```python
from build123d import *

# Parameters (mm, degrees)
SKETCH1_R           = 6.35
SKETCH1_W           = 38.1
SKETCH1_H           = 13.818872092
BOSS_EXTRUDE1_DEPTH = 12.7


with BuildPart() as part:
    # Sketch1 → Boss-Extrude1 (new body)
    # profile 1 of 2: a face of its own
    with BuildSketch(Plane.XY):
        with BuildLine():
            Line((129.803523023, 13.72866743), (129.803523023, 32.77866743))
            Line((129.803523023, 32.77866743), (104.403523023, 32.77866743))
            Line((104.403523023, 32.77866743), (89.290523023, 32.77866743))
            Line((89.290523023, 32.77866743), (51.190523023, 32.77866743))
            Line((51.190523023, 32.77866743), (44.078523023, 32.77866743))
            Line((44.078523023, 32.77866743), (42.173523023, 32.77866743))
            ThreePointArc((42.173523023, 32.77866743), (0.864344867, 49.889489273), (-16.246476977, 91.19866743))
            Line((-16.246476977, 91.19866743), (-16.246476977, 115.32866743))
            Line((-16.246476977, 115.32866743), (-18.528129693, 124.368857105))
            ThreePointArc((-18.528129693, 124.368857105), (-35.296476977, 134.37866743), (-52.064824261, 124.368857105))
            Line((-52.064824261, 124.368857105), (-54.346476977, 115.32866743))
            Line((-54.346476977, 115.32866743), (-54.346476977, 91.438289009))
            ThreePointArc((-54.346476977, 91.438289009), (-63.850433524, 50.845698757), (-90.386686587, 18.691214671))
            Line((-90.386686587, 18.691214671), (-171.948476977, -43.42133257))
            Line((-171.948476977, -43.42133257), (-87.747476977, -43.42133257))
            Line((-87.747476977, -43.42133257), (-87.747476977, -49.77133257))
            Line((-87.747476977, -49.77133257), (-61.229320991, -49.77133257))
            Line((-61.229320991, -49.77133257), (-16.694588765, -49.77133257))
            Line((-16.694588765, -49.77133257), (64.652523023, -49.77133257))
            Line((64.652523023, -49.77133257), (64.652523023, -43.42133257))
            Line((64.652523023, -43.42133257), (129.803523023, -43.42133257))
            Line((129.803523023, -43.42133257), (129.803523023, -24.37133257))
            Line((129.803523023, -24.37133257), (139.328523023, -24.37133257))
            Line((139.328523023, -24.37133257), (139.328523023, 13.72866743))
            Line((139.328523023, 13.72866743), (129.803523023, 13.72866743))
        make_face()
        with Locations((-35.296476977, 115.32866743)):
            Circle(SKETCH1_R, mode=Mode.SUBTRACT)
    # profile 2 of 2: a face of its own
    with BuildSketch(Plane.XY):
        with Locations((70.240523023, 39.688103476)):
            Rectangle(SKETCH1_W, SKETCH1_H)
    extrude(amount=BOSS_EXTRUDE1_DEPTH)


solid = part.part
```
For this review, take the finished solid that the model builds, in its own axes (mm). A direction names the side the tool comes from. Give positions to 0.01 mm unless a question says otherwise; leave off trailing zeros. Order: outer loops, then holes, each group sorted by start corner. A loop starts at its lowest first (then second) coordinate and runs counter-clockwise, first axis right, second up.
1) For faces 1 (the face through (47, 32.779, 6)), 2 (the face through (135, 13.729, 6)), 3 (the face through (-54.346, 104, 6)), 4 (the face through (129.804, -34, 6)), list the 3-axis set-ups (+Z, -Z, +X, -X, +Y, -Y) from which the entire face can be reached by the end or side of a thin tool; tool diameter is ignored.
2) Insertion check: pin 1 (4 mm diameter, centred on x = 71.5, z = 7.5, fed in from +Y); pin 2 (7 mm diameter, centred on x = 45, z = 8, fed in from +Y); pin 3 (3 mm diameter, centred on y = -45.5, z = 3.5, fed in from +X); pin 4 (11.5 mm diameter, centred on x = -35.3, y = 115.33, fed in from +Z). Each pin has a flat end and moves straight along its axis. Give the tip position at first contact, or say it passes through.
3) Take a section at D-D (x = -72.5). Give the boundary of the cut face in (y, z).
4) Take a section at C-C (y = 98). Give the boundary of the cut face in (x, z), then the cut area to 3 significant figures.
5) The part is to be moulded in two halves that separate along X. For faces 5 (the face through (-53.19, 119.91, 6.26)), 6 (the face through (-36.67, 109.13, 6.26)), 7 (the face through (89.291, 40, 6)), say which applies: released by +X, released by -X, zero draft, split by the parting line, or undercut.
6) Take a section at B-B (x = -34). Give the boundary of the cut face in (y, z), then the cut area to 3 significant figures.
7) Wall thickness on line 1 (X direction, y = 117.5, z = 9); line 2 (Y direction, x = 105, z = 1.25); line 3 (X direction, y = 91.5, z = 5): over which ranges is each line inside the solid? List them lowest first.
8) Take a section at A-A (z = 2.75). Give the boundary of the cut face in (x, y), then the cut area to 3 significant figures.
Derived:
1. face 1: +Z, -Z, +Y
1. face 2: +Z, -Z, +X, +Y
1. face 3: +Z, -Z, -X, +Y
1. face 4: +Z, -Z, +X, -Y
2. pin 1: stops at y = 46.6
2. pin 2: stops at y = 32.78
2. pin 3: stops at x = 64.65
2. pin 4: passes through
3. outline: (-49.77, 0) - (36.75, 0) - (36.75, 12.7) - (-49.77, 12.7) - close
4. outline: (-54.35, 0) - (-16.25, 0) - (-16.25, 12.7) - (-54.35, 12.7) - close
4. area: 484 mm2
5. face 5: released by -X
5. face 6: undercut
5. face 7: released by +X
6. outline: (-49.77, 0) - (109.11, 0) - (109.11, 12.7) - (-49.77, 12.7) - close; (121.54, 0) - (134.33, 0) - (134.33, 12.7) - (121.54, 12.7) - close
6. area: 2,180 mm2
7. line 1: x = -53.8 to -41.26, -29.33 to -16.79
7. line 2: y = -43.42 to 32.78
7. line 3: x = -54.35 to -16.25
8. outline: (-171.95, -43.42) - (-87.75, -43.42) - (-87.75, -49.77) - (64.65, -49.77) - (64.65, -43.42) - (129.8, -43.42) - (129.8, -24.37) - (139.33, -24.37) - (139.33, 13.73) - (129.8, 13.73) - (129.8, 32.78) - (89.29, 32.78) - (89.29, 46.6) - (51.19, 46.6) - (51.19, 32.78) - (42.17, 32.78) arc R58.42 cw to (-16.25, 91.2) - (-16.25, 115.33) - (-18.53, 124.37) arc R19.05 ccw to (-52.06, 124.37) - (-54.35, 115.33) - (-54.35, 91.44) arc R91.44 cw to (-90.39, 18.69) - close; hole circle Ø12.7 at (-35.3, 115.33)
8. area: 25,800 mm2
